```python
from build123d import *

# Parameters (mm, degrees)
SKETCH_1_R          = 210
SKETCH_1_R_2        = 203
EXTRUDE_2_DEPTH     = 174
EXTRUDE_START       = -174
EXTRUDE_4_DEPTH     = 174
CUT_EXTRUDE_1_DEPTH = 654
EXTRUDE_5_DEPTH     = 174
EXTRUDE_6_DEPTH     = 174
EXTRUDE_7_DEPTH     = 174
EXTRUDE_8_DEPTH     = 174
CUT_EXTRUDE_START   = -654
CUT_EXTRUDE_2_DEPTH = 654
SKETCH_10_W         = 20.487801248
SKETCH_10_H         = 174
CUT_EXTRUDE_3_DEPTH = 327
SKETCH_11_W         = 235.63772895
SKETCH_11_H         = 249.192111589
CUT_EXTRUDE_4_DEPTH = 238


with BuildPart() as part:
    # 草图1 → 凸台-拉伸2 (new body)
    with BuildSketch(Plane.XY):
        Circle(SKETCH_1_R)
        Circle(SKETCH_1_R_2, mode=Mode.SUBTRACT)
    extrude(amount=EXTRUDE_2_DEPTH)

    # 草图2 → 凸台-拉伸4 (add)
    with BuildSketch(Plane.XY.offset(174).offset(EXTRUDE_START)):
        with BuildLine():
            Line((-170.735431044, -102), (-173.735431044, -102))
            Line((-173.735431044, -102), (-175.513532242, -102))
            ThreePointArc((-175.513532242, -102), (-174.63092392, -103.50381834), (-173.735431044, -105))
            Line((-173.735431044, -105), (-170.735431044, -105))
            Line((-170.735431044, -105), (-170.735431044, -102))
        make_face()
        with BuildLine():
            ThreePointArc((173.735431044, -105), (174.63092392, -103.50381834), (175.513532242, -102))
            Line((175.513532242, -102), (173.735431044, -102))
            Line((173.735431044, -102), (170.735431044, -102))
            Line((170.735431044, -102), (170.735431044, -105))
            Line((170.735431044, -105), (173.735431044, -105))
        make_face()
    extrude(amount=EXTRUDE_4_DEPTH)

    # 草图3 → 切除-拉伸1 (cut)
    with BuildSketch(Plane.XY.offset(174)):
        Polygon((-170.735431044, -102), (238.333646515, -102), (254.334169784, 272.292523591), (-334.569415043, 221.85110305), (-306.830562533, -102), align=None)
    extrude(amount=-CUT_EXTRUDE_1_DEPTH, mode=Mode.SUBTRACT)

    # 草图5 → 凸台-拉伸5 (add)
    with BuildSketch(Plane.XY.offset(174).offset(EXTRUDE_START)):
        with BuildLine():
            Line((-120, -209.75), (-10.243900624, -209.75))
            ThreePointArc((-10.243900624, -209.75), (-67.755470707, -198.769203322), (-120, -172.336879396))
            Line((-120, -172.336879396), (-120, -209.75))
        make_face()
        with BuildLine():
            ThreePointArc((120, -172.336879396), (67.755470707, -198.769203322), (10.243900624, -209.75))
            Line((10.243900624, -209.75), (120, -209.75))
            Line((120, -209.75), (120, -172.336879396))
        make_face()
    extrude(amount=EXTRUDE_5_DEPTH)

    # 草图6 → 凸台-拉伸6 (add)
    with BuildSketch(Plane.XY.offset(174).offset(EXTRUDE_START)):
        with BuildLine():
            Line((-175.513532242, -102), (-166.195667814, -102))
            ThreePointArc((-166.195667814, -102), (0, -195), (166.195667814, -102))
            Line((166.195667814, -102), (175.513532242, -102))
            ThreePointArc((175.513532242, -102), (0, -203), (-175.513532242, -102))
        make_face()
    extrude(amount=EXTRUDE_6_DEPTH)

    # 草图7 → 凸台-拉伸7 (add)
    with BuildSketch(Plane.XY.offset(174).offset(EXTRUDE_START)):
        with BuildLine():
            Line((-166.933126535, -92), (-166.933126535, -95))
            Line((-166.933126535, -95), (-170.293863659, -95))
            ThreePointArc((-170.293863659, -95), (0, -195), (170.293863659, -95))
            Line((170.293863659, -95), (166.933126535, -95))
            Line((166.933126535, -95), (166.933126535, -92))
            Line((166.933126535, -92), (171.933126535, -92))
            Line((171.933126535, -92), (188.496850106, -92))
            ThreePointArc((188.496850106, -92), (0, -209.75), (-188.496850106, -92))
            Line((-188.496850106, -92), (-171.933126535, -92))
            Line((-171.933126535, -92), (-166.933126535, -92))
        make_face()
    extrude(amount=EXTRUDE_7_DEPTH)

    # 草图8 → 凸台-拉伸8 (add)
    with BuildSketch(Plane(origin=(0, 0, 0), x_dir=(-1, 0, 0), z_dir=(0, 0, -1))):
        with BuildLine():
            Line((166.933126535, -92), (163.933126535, -92))
            Line((163.933126535, -92), (163.933126535, -99))
            Line((163.933126535, -99), (168, -99))
            ThreePointArc((168, -99), (169.158755456, -97.006780447), (170.293863659, -95))
            Line((170.293863659, -95), (166.933126535, -95))
            Line((166.933126535, -95), (166.933126535, -92))
        make_face()
        with BuildLine():
            Line((-166.933126535, -95), (-170.293863659, -95))
            ThreePointArc((-170.293863659, -95), (-169.158755456, -97.006780447), (-168, -99))
            Line((-168, -99), (-163.933126535, -99))
            Line((-163.933126535, -99), (-163.933126535, -92))
            Line((-163.933126535, -92), (-166.933126535, -92))
            Line((-166.933126535, -92), (-166.933126535, -95))
        make_face()
    extrude(amount=-EXTRUDE_8_DEPTH)

    # 草图9 → 切除-拉伸2 (cut)
    with BuildSketch(Plane.XY.offset(174).offset(CUT_EXTRUDE_START)):
        with BuildLine():
            Line((0, -195), (0, -182.225251044))
            Line((0, -182.225251044), (-50, -182.225251044))
            Line((-50, -182.225251044), (-50, -188.48076825))
            ThreePointArc((-50, -188.48076825), (-25.211606368, -193.363323576), (0, -195))
        make_face()
        with BuildLine():
            Line((0, -209.75), (0, -195))
            ThreePointArc((0, -195), (-25.211606368, -193.363323576), (-50, -188.48076825))
            Line((-50, -188.48076825), (-50, -195))
            Line((-50, -195), (-50, -209.75))
            Line((-50, -209.75), (-10.243900624, -209.75))
            Line((-10.243900624, -209.75), (0, -209.75))
        make_face()
        with BuildLine():
            ThreePointArc((50, -188.48076825), (25.211606368, -193.363323576), (0, -195))
            Line((0, -195), (0, -209.75))
            Line((0, -209.75), (10.243900624, -209.75))
            Line((10.243900624, -209.75), (50, -209.75))
            Line((50, -209.75), (50, -195))
            Line((50, -195), (50, -188.48076825))
        make_face()
        with BuildLine():
            Line((50, -182.225251044), (0, -182.225251044))
            Line((0, -182.225251044), (0, -195))
            ThreePointArc((0, -195), (25.211606368, -193.363323576), (50, -188.48076825))
            Line((50, -188.48076825), (50, -182.225251044))
        make_face()
    extrude(amount=CUT_EXTRUDE_2_DEPTH, mode=Mode.SUBTRACT)


with BuildPart() as cut_extrude_2_piece_1:
    # of the separate pieces the step leaves, piece 1, a body of its own (cut_extrude_2_pieces)
    add(part.part.solids().sort_by_distance((-183.564702489, -102, 0))[0])

    # 草图11 → 切除-拉伸4 (cut)
    with BuildSketch(Plane(origin=(0, 0, 0), x_dir=(-1, 0, 0), z_dir=(0, 0, -1))):
        with Locations((136.586471206, -141.23053543)):
            Rectangle(SKETCH_11_W, SKETCH_11_H)
    extrude(amount=-CUT_EXTRUDE_4_DEPTH, mode=Mode.SUBTRACT)


with BuildPart() as cut_extrude_2_piece_2:
    # of the separate pieces the step leaves, piece 2, a body of its own (cut_extrude_2_pieces)
    add(part.part.solids().sort_by_distance((50, -188.48076825, 0))[0])


with BuildPart() as cut_extrude_2_piece_3:
    # of the separate pieces the step leaves, piece 3, a body of its own (cut_extrude_2_pieces)
    add(part.part.solids().sort_by_distance((10.243900624, -209.75, 0))[0])

    # 草图10 → 切除-拉伸3 (cut, symmetric)
    with BuildSketch(Plane(origin=(0, -209.75, 0), x_dir=(1, 0, 0), z_dir=(0, 1, 0))):
        with Locations((0, -87)):
            Rectangle(SKETCH_10_W, SKETCH_10_H)
    extrude(amount=CUT_EXTRUDE_3_DEPTH, both=True, mode=Mode.SUBTRACT)


solid = cut_extrude_2_piece_2.part
```
Source: CAD feature listing. Evaluate the final solid. Frame: model axes, mm. A direction names the side the tool comes from. Coordinates: 2 decimals unless noted, no trailing zeros. Write each loop counter-clockwise with the first axis right and the second up, starting at its lowest first coordinate (ties: lowest second). Pieces come first, ordered by that corner, then holes. Notation, with made-up numbers: (58.5, -15) - (84.5, -15) arc R36 ccw to (84.5, 22) - close; hole circle Ø3 at (26.25, 89). An arc over 180 degrees is marked (long way). Answer as a JSON object with one key per item and string values.
Q1. Section query B-B, the plane y = -196. Output: boundary loops of the cut face in (x, z), plus the area to 3 significant figures.
Ans:
{"outline": "(50, 0) - (120, 0) - (120, 174) - (50, 174) - close", "area": "12,200 mm2"}
Q2. Set-up query: faces 1 (the flat face through (163.933, -96, 86)), 2 (the flat face through (50, -199, 86)), 3 (the flat face through (120, -191, 86)). Return all of +Z, -Z, +X, -X, +Y, -Y with unobstructed straight access to the full face (end or side cutting, diameter ignored); none if empty.
Ans:
{"face 1": "+Z, -Z, -X, +Y", "face 2": "+Z, -Z, -X, +Y, -Y", "face 3": "+Z, -Z, +X, -Y"}
Q3. First-contact query: pin 1 Ø4 at (x, y) = (112.5, -154.5) entering from -Z; pin 2 Ø4.5 at (x, z) = (166, 55) entering from -Y; pin 3 Ø8 at (x, z) = (100, 104) entering from +Y; pin 4 Ø2 at (x, z) = (158.5, 153.5) entering from -Y. Flat tips, straight axial feed; report the tip coordinate or a pass-through.
Ans:
{"pin 1": "passes through", "pin 2": "stops at y = -131.48", "pin 3": "stops at y = -164.95", "pin 4": "stops at y = -138.9"}
Q4. Draft query along Y for faces 4 (the flat face through (114, -172, 174)), 5 (the flat face through (176, -92, 86)), 6 (the flat face through (166, -99, 86)). Return one class per face: released by +Y, released by -Y, zero draft, split by the parting line, or undercut.
Ans:
{"face 4": "zero draft", "face 5": "released by +Y", "face 6": "undercut"}
Q5. Material intervals for line 1 (X direction, y = -199.5, z = 93); line 2 (X direction, y = -98, z = 32.5); line 3 (Y direction, x = 138.5, z = 160), sorted ascending. Write a range as [from, to].
Ans:
{"line 1": "x = [50, 120]", "line 2": "x = [163.93, 185.45]", "line 3": "y = [-157.85, -137.27]"}
Q6. Section query C-C, the plane x = 128. Output: boundary loops of the cut face in (y, z), plus the area to 3 significant figures.
Ans:
{"outline": "(-166.48, 0) - (-147.11, 0) - (-147.11, 174) - (-166.48, 174) - close", "area": "3,370 mm2"}
Q7. Section query A-A, the plane z = 105.5. Output: boundary loops of the cut face in (x, y), plus the area to 3 significant figures.
Ans:
{"outline": "(50, -209.75) - (120, -209.75) - (120, -172.34) arc R210 ccw to (183.56, -102) - (183.28, -102) arc R209.75 ccw to (188.5, -92) - (163.93, -92) - (163.93, -99) - (168, -99) arc R195 cw to (50, -188.48) - close", "area": "3,950 mm2"}
